```python
from build123d import *

# Parameters (mm, degrees)
BOSS_EXTRUDE1_DEPTH  = 8
SKETCH2_R            = 1.624765057
CUT_EXTRUDE1_DEPTH   = 6
CHAMFER1_SIZE        = 0.5
SKETCH3_W            = 32.228932188
SKETCH3_H            = 1
CUT_EXTRUDE2_DEPTH   = 48.964700562
SKETCH4_W            = 32.228932188
SKETCH4_H            = 1
CUT_EXTRUDE3_DEPTH   = 48.964700562
CUT_EXTRUDE4_DEPTH   = 1
MIRROR2_COPY_1_DEPTH = 1
BOSS_EXTRUDE2_DEPTH  = 24
BOSS_EXTRUDE4_DEPTH  = 8
SKETCH22_W           = 16
SKETCH22_H           = 2.5
BOSS_EXTRUDE5_DEPTH  = 6.5
CHAMFER3_SIZE        = 0.5
SKETCH23_W           = 15.8
SKETCH23_H           = 6.4
CUT_EXTRUDE5_DEPTH   = 1.9
SKETCH24_R           = 12.5
CUT_EXTRUDE6_DEPTH   = 0.75
SKETCH25_R           = 6
BOSS_EXTRUDE6_DEPTH  = 2
SKETCH26_R           = 2.25
CUT_EXTRUDE7_DEPTH   = 5
SKETCH27_R           = 1.25207439
BOSS_EXTRUDE7_DEPTH  = 27
CHAMFER5_SIZE        = 0.25
FILLET1_R            = 2
FILLET3_R            = 1
FILLET4_R            = 1


with BuildPart() as part:
    # Sketch1 → Boss-Extrude1 (new body)
    with BuildSketch(Plane(origin=(0, 0, 0), x_dir=(1, 0, 0), z_dir=(0, 1, 0))):
        Polygon((-21.15, -17.614466094), (-21.15, 17.614466094), (-17.614466094, 21.15), (17.614466094, 21.15), (21.15, 17.614466094), (21.15, -17.614466094), (17.614466094, -21.15), (-17.614466094, -21.15), align=None)
    extrude(amount=-BOSS_EXTRUDE1_DEPTH)

    # Sketch2 → Cut-Extrude1 (cut)
    with BuildSketch(Plane(origin=(0, 0, 0), x_dir=(1, 0, 0), z_dir=(0, 1, 0))):
        with Locations(Location((-15.5, 15.5, 0), (0, 0, 270))):
            Circle(SKETCH2_R)
        with Locations(Location((15.5, 15.5, 0), (0, 0, 90))):
            Circle(SKETCH2_R)
        with Locations(Location((15.5, -15.5, 0), (0, 0, 270))):
            Circle(SKETCH2_R)
        with Locations(Location((-15.5, -15.5, 0), (0, 0, 90))):
            Circle(SKETCH2_R)
    extrude(amount=-CUT_EXTRUDE1_DEPTH, mode=Mode.SUBTRACT)

    # Chamfer1
    chamfer1_edges = [part.edges().sort_by_distance(p)[0] for p in [
        (21.15, 0, 0),
        (19.382233047, 0, 19.382233047),
        (0, 0, 21.15),
        (-19.382233047, 0, 19.382233047),
        (-21.15, 0, 0),
        (-19.382233047, 0, -19.382233047),
        (0, 0, -21.15),
        (19.382233047, 0, -19.382233047),
    ]]
    chamfer(chamfer1_edges, length=CHAMFER1_SIZE)

    # Sketch3 → Cut-Extrude2 (cut, through all)
    with BuildSketch(Plane(origin=(21.15, 0, 0), x_dir=(0, 0, -1), z_dir=(1, 0, 0))):
        with Locations((0, -7.5)):
            Rectangle(SKETCH3_W, SKETCH3_H)
    extrude(amount=-CUT_EXTRUDE2_DEPTH, mode=Mode.SUBTRACT)

    # Sketch4 → Cut-Extrude3 (cut, through all)
    with BuildSketch(Plane.XY.offset(21.15)):
        with Locations((0, -7.5)):
            Rectangle(SKETCH4_W, SKETCH4_H)
    extrude(amount=-CUT_EXTRUDE3_DEPTH, mode=Mode.SUBTRACT)

    # Sketch5 → Cut-Extrude4 (cut)
    with BuildSketch(Plane.XZ.offset(8)):
        Polygon((-21.15, 16.114466094), (-16.114466094, 21.15), (-16.114466094, 16.114466094), align=None)
    cut_extrude4 = extrude(amount=-CUT_EXTRUDE4_DEPTH, mode=Mode.SUBTRACT)

    # Mirror1: Cut-Extrude4 across plane
    add(cut_extrude4.mirror(Plane(origin=(0, 0, 0), x_dir=(0, 0, 1), z_dir=(1, 0, 0))), mode=Mode.SUBTRACT)

    # Mirror2: Cut-Extrude4 across plane
    add(cut_extrude4.mirror(Plane.XY), mode=Mode.SUBTRACT)

    # Mirror2 copy 1 sketch → Mirror2 copy 1 (cut)
    with BuildSketch(Plane(origin=(0, -8, 0), x_dir=(-1, 0, 0), z_dir=(0, -1, 0))):
        Polygon((-21.15, 16.114466094), (-16.114466094, 21.15), (-16.114466094, 16.114466094), align=None)
    extrude(amount=-MIRROR2_COPY_1_DEPTH, mode=Mode.SUBTRACT)

    # Sketch6 → Boss-Extrude2 (add)
    with BuildSketch(Plane.XZ.offset(7)):
        Polygon((-21.15, -16.114466094), (-21.15, 16.114466094), (-16.114466094, 21.15), (16.114466094, 21.15), (21.15, 16.114466094), (21.15, -16.114466094), (16.114466094, -21.15), (-16.114466094, -21.15), align=None)
    extrude(amount=BOSS_EXTRUDE2_DEPTH)

    # Sketch16 → Boss-Extrude4 (add)
    with BuildSketch(Plane.XZ.offset(31)):
        Polygon((-21.15, -17.614466094), (-21.15, 17.614466094), (-17.614466094, 21.15), (17.614466094, 21.15), (21.15, 17.614466094), (21.15, -17.614466094), (17.614466094, -21.15), (-17.614466094, -21.15), align=None)
    extrude(amount=BOSS_EXTRUDE4_DEPTH)

    # Sketch22 → Boss-Extrude5 (add)
    with BuildSketch(Plane.XY.offset(21.15)):
        with Locations((0, -37.75)):
            Rectangle(SKETCH22_W, SKETCH22_H)
    extrude(amount=BOSS_EXTRUDE5_DEPTH)

    # Chamfer3
    chamfer3_edges = [part.edges().sort_by_distance(p)[0] for p in [
        (-19.382233047, -39, -19.382233047),
        (0, -39, -21.15),
        (19.382233047, -39, -19.382233047),
        (21.15, -39, 0),
        (19.382233047, -39, 19.382233047),
        (12.807233047, -39, 21.15),
        (-19.382233047, -39, 19.382233047),
        (-21.15, -39, 0),
        (-12.807233047, -39, 21.15),
        (-8, -39, 24.4),
        (8, -39, 24.4),
        (0, -39, 27.65),
    ]]
    chamfer(chamfer3_edges, length=CHAMFER3_SIZE)

    # Sketch23 → Cut-Extrude5 (cut)
    with BuildSketch(Plane(origin=(0, -36.5, 0), x_dir=(1, 0, 0), z_dir=(0, 1, 0))):
        with Locations((0, -24.35)):
            Rectangle(SKETCH23_W, SKETCH23_H)
    extrude(amount=-CUT_EXTRUDE5_DEPTH, mode=Mode.SUBTRACT)

    # Sketch24 → Cut-Extrude6 (cut)
    with BuildSketch(Plane(origin=(0, 0, 0), x_dir=(1, 0, 0), z_dir=(0, 1, 0))):
        with Locations(Location((0, 0, 0), (0, 0, 270))):
            Circle(SKETCH24_R)
    extrude(amount=-CUT_EXTRUDE6_DEPTH, mode=Mode.SUBTRACT)

    # Sketch25 → Boss-Extrude6 (add)
    with BuildSketch(Plane(origin=(0, -0.75, 0), x_dir=(1, 0, 0), z_dir=(0, 1, 0))):
        with Locations(Location((0, 0, 0), (0, 0, 270))):
            Circle(SKETCH25_R)
    extrude(amount=BOSS_EXTRUDE6_DEPTH)

    # Sketch26 → Cut-Extrude7 (cut)
    with BuildSketch(Plane(origin=(0, 1.25, 0), x_dir=(1, 0, 0), z_dir=(0, 1, 0))):
        with Locations(Location((0, 0, 0), (0, 0, 270))):
            Circle(SKETCH26_R)
    extrude(amount=-CUT_EXTRUDE7_DEPTH, mode=Mode.SUBTRACT)

    # Sketch27 → Boss-Extrude7 (add)
    with BuildSketch(Plane(origin=(0, -3.75, 0), x_dir=(1, 0, 0), z_dir=(0, 1, 0))):
        with Locations(Location((0, 0, 0), (0, 0, 270))):
            Circle(SKETCH27_R)
    extrude(amount=BOSS_EXTRUDE7_DEPTH)

    # Chamfer5
    chamfer5_edges = [part.edges().sort_by_distance(p)[0] for p in [
        (0, 23.25, -1.25207439),
    ]]
    chamfer(chamfer5_edges, length=CHAMFER5_SIZE)

    # Fillet1
    fillet1_edges = [part.edges().sort_by_distance(p)[0] for p in [
        (-21.15, -19.5, -16.114466094),
        (-16.114466094, -19.5, -21.15),
        (16.114466094, -19.5, -21.15),
        (21.15, -19.5, -16.114466094),
        (21.15, -19.5, 16.114466094),
        (16.114466094, -19.5, 21.15),
        (-16.114466094, -19.5, 21.15),
        (-21.15, -19.5, 16.114466094),
    ]]
    fillet(fillet1_edges, radius=FILLET1_R)

    # Fillet3
    fillet3_edges = [part.edges().sort_by_distance(p)[0] for p in [
        (-21.15, -4.25, 17.614466094),
        (-21.15, -4.25, -17.614466094),
        (-17.614466094, -4.25, -21.15),
        (17.614466094, -4.25, -21.15),
        (21.15, -4.25, -17.614466094),
        (21.15, -4.25, 17.614466094),
        (17.614466094, -4.25, 21.15),
        (-17.614466094, -4.25, 21.15),
    ]]
    fillet(fillet3_edges, radius=FILLET3_R)

    # Fillet4
    fillet4_edges = [part.edges().sort_by_distance(p)[0] for p in [
        (-21.15, -34.75, -17.614466094),
        (-21.15, -34.75, 17.614466094),
        (-17.614466094, -34.75, 21.15),
        (17.614466094, -34.75, 21.15),
        (21.15, -34.75, 17.614466094),
        (21.15, -34.75, -17.614466094),
        (17.614466094, -34.75, -21.15),
        (-17.614466094, -34.75, -21.15),
    ]]
    fillet(fillet4_edges, radius=FILLET4_R)


solid = part.part
```
Could you check a few things on this model? Use its own coordinates, in mm. A direction names the side the tool comes from. Coordinates: 2 decimals unless noted, no trailing zeros. Loops run counter-clockwise (first coordinate to the right, second up) from the corner with the lowest first, then second, coordinate; pieces in that order, holes last. Notation, with made-up numbers: M -1.75,41.5 L 24.25,41.5 A19 cw 24.25,58.5 Z; hole C 35,-15 d7. An arc over 180 degrees is marked long. Put each result on its own line as item: value. Start each with the question number.
(1) Thinking about a two-plate mould opening in Z: for faces 5 (the face through (-19.362, -4.198, 19.403)), 6 (the face through (19, -31, 19)), 7 (the face through (0.376, 9.438, 1.194)), which applies, pulls with the +Z half, pulls with the -Z half, needs draft (parallel to the pull), parting line crosses it, or undercut?
(2) I need wall thicknesses on line 1 (X direction, y = -2.8, z = -15.5); line 2 (X direction, y = -0.65, z = 0); line 3 (Z direction, x = 8, y = -22.5). Which ranges of each line are inside material? Lowest first, please. Write a range as from..to.
(3) Suppose I cut it at D-D on z = -11. Please give me the cut outline in (x, y), then the cut area to 3 significant figures.
(4) For faces 1 (the face through (-19, -8, 19)), 2 (the face through (0, -38.4, 24)), 3 (the face through (-21.002, -19.661, -16.041)), 4 (the face through (19, -31, -19)), which set-ups out of +Z, -Z, +X, -X, +Y, -Y let a thin tool reach every point of the face, with its end or its side?
(5) Will these pins go through, and if not, where does the flat tip stop? P1, Ø12, axis at y = 16.5, z = 1, coming from the +X side; P2, Ø7, axis at x = 1, z = 24, coming from the +Y side; P3, Ø5, axis at x = -9.5, y = -8, coming from the +Z side.
(6) Suppose I cut it at A-A on z = 0. Please give me the cut outline in (x, y).
(7) Suppose I cut it at C-C on y = -16. Please give me the cut outline in (x, z).
Solutions:
1. face 5: pulls with the +Z half
1. face 6: needs draft
1. face 7: undercut
2. line 1: x = -21.15..-17.12, -13.88..13.88, 17.12..21.15
2. line 2: x = -21.15..-12.5, -6..-2.25, -1.25..1.25, 2.25..6, 12.5..21.15
2. line 3: z = -21.15..21.15
3. outline: M -21.15,-38.5 L -20.65,-39 L 20.65,-39 L 21.15,-38.5 L 21.15,-0.5 L 20.65,0 L 5.94,0 L 5.94,-0.75 L -5.94,-0.75 L -5.94,0 L -20.65,0 L -21.15,-0.5 Z
3. area: 1,640 mm2
4. face 1: +Z, -X
4. face 2: +Y
4. face 3: -Z, -X
4. face 4: -Z, +X
5. P1: stops at x = 1.25
5. P2: stops at y = 0
5. P3: stops at z = 21.15
6. outline: M -21.15,-38.5 L -20.65,-39 L 20.65,-39 L 21.15,-38.5 L 21.15,-0.5 L 20.65,0 L 12.5,0 L 12.5,-0.75 L 6,-0.75 L 6,1.25 L 2.25,1.25 L 2.25,-3.75 L 1.25,-3.75 L 1.25,23 L 1,23.25 L -1,23.25 L -1.25,23 L -1.25,-3.75 L -2.25,-3.75 L -2.25,1.25 L -6,1.25 L -6,-0.75 L -12.5,-0.75 L -12.5,0 L -20.65,0 L -21.15,-0.5 Z
7. outline: M -21.15,-15.29 A2 ccw -20.56,-16.7 L -16.7,-20.56 A2 ccw -15.29,-21.15 L 15.29,-21.15 A2 ccw 16.7,-20.56 L 20.56,-16.7 A2 ccw 21.15,-15.29 L 21.15,15.29 A2 ccw 20.56,16.7 L 16.7,20.56 A2 ccw 15.29,21.15 L -15.29,21.15 A2 ccw -16.7,20.56 L -20.56,16.7 A2 ccw -21.15,15.29 Z
